from build123d import *

# Parameters (mm, degrees)
SKETCH_W        = 115
SKETCH_H        = 62
SKETCH_R        = 1.75
PAD_DEPTH       = 5
FILLET_R        = 1
FILLET001_R     = 1
FILLET002_R     = 3
PAD001_DEPTH    = 40
SKETCH002_W     = 95
SKETCH002_H     = 62
PAD002_DEPTH    = 3
FILLET003_R     = 3
FILLET004_R     = 1
SKETCH003_W     = 40
SKETCH003_H     = 15
POCKET_DEPTH    = 5
SKETCH004_R     = 1.75
POCKET001_DEPTH = 5
FILLET005_R     = 4
POCKET002_DEPTH = 5
SKETCH006_W     = 95
SKETCH006_H     = 43
POCKET003_DEPTH = 1
SKETCH007_W     = 95
SKETCH007_H     = 43
PAD003_DEPTH    = 1
PAD004_DEPTH    = 1
FILLET006_R     = 1


with BuildPart() as part:
    # Sketch → Pad (new body)
    with BuildSketch(Plane.XY):
        Rectangle(SKETCH_W, SKETCH_H)
        with Locations((-50, 22.5)):
            Circle(SKETCH_R, mode=Mode.SUBTRACT)
        with Locations((50, 22.5)):
            Circle(SKETCH_R, mode=Mode.SUBTRACT)
        with Locations((-50, -22.5)):
            Circle(SKETCH_R, mode=Mode.SUBTRACT)
        with Locations((50, -22.5)):
            Circle(SKETCH_R, mode=Mode.SUBTRACT)
        with BuildLine():
            ThreePointArc((-40.5, 15), (-42.62132, 14.12132), (-43.5, 12))
            Line((-43.5, -12), (-43.5, 12))
            ThreePointArc((-43.5, -12), (-42.62132, -14.12132), (-40.5, -15))
            Line((-40.5, -15), (-31.5, -15))
            ThreePointArc((-31.5, -15), (-29.37868, -14.12132), (-28.5, -12))
            Line((-28.5, 12), (-28.5, -12))
            ThreePointArc((-28.5, 12), (-29.37868, 14.12132), (-31.5, 15))
            Line((-40.5, 15), (-31.5, 15))
        make_face(mode=Mode.SUBTRACT)
    extrude(amount=PAD_DEPTH)

    # Fillet
    fillet_edges = [part.edges().sort_by_distance(p)[0] for p in [
        (-36, -15, 0),
        (-29.37868, -14.12132, 0),
        (-28.5, 0, 0),
        (-42.62132, -14.12132, 0),
        (-43.5, 0, 0),
        (-42.62132, 14.12132, 0),
        (-36, 15, 0),
        (-29.37868, 14.12132, 0),
    ]]
    fillet(fillet_edges, radius=FILLET_R)

    # Fillet001
    fillet001_edges = [part.edges().sort_by_distance(p)[0] for p in [
        (-43.5, 0, 5),
        (-42.62132, -14.12132, 5),
        (-36, -15, 5),
        (-29.37868, -14.12132, 5),
        (-28.5, 0, 5),
        (-29.37868, 14.12132, 5),
        (-36, 15, 5),
        (-42.62132, 14.12132, 5),
    ]]
    fillet(fillet001_edges, radius=FILLET001_R)

    # Fillet002
    fillet002_edges = [part.edges().sort_by_distance(p)[0] for p in [
        (-57.5, -31, 2.5),
        (-57.5, 31, 2.5),
        (57.5, -31, 2.5),
        (57.5, 31, 2.5),
    ]]
    fillet(fillet002_edges, radius=FILLET002_R)

    # Sketch001 (on Face1 of Fillet002) → Pad001 (join)
    with BuildSketch(Plane.XY.offset(5)):
        Polygon((-47.5, 31), (47.5, 31), (47.5, -31), (45.5, -31), (45.5, 29), (-45.5, 29), (-45.5, -31), (-47.5, -31), align=None)
    extrude(amount=PAD001_DEPTH)

    # Sketch002 (on Face15 of Pad001) → Pad002 (join)
    with BuildSketch(Plane.XY.offset(45)):
        Rectangle(SKETCH002_W, SKETCH002_H)
    extrude(amount=PAD002_DEPTH)

    # Fillet003
    fillet003_edges = [part.edges().sort_by_distance(p)[0] for p in [
        (-45.5, 29, 25),
        (45.5, 29, 25),
    ]]
    fillet(fillet003_edges, radius=FILLET003_R)

    # Fillet004
    fillet004_edges = [part.edges().sort_by_distance(p)[0] for p in [
        (-47.5, 31, 25),
        (-45.5, -2.5, 45),
        (-44.62132, 28.12132, 45),
        (0, 29, 45),
        (44.62132, 28.12132, 45),
        (45.5, -2.5, 45),
    ]]
    fillet(fillet004_edges, radius=FILLET004_R)

    # Sketch003 (on Face21 of Fillet004) → Pocket (cut)
    with BuildSketch(Plane(origin=(-47.5, 0, 0), x_dir=(0, -1, 0), z_dir=(-1, 0, 0))):
        with Locations((0, 15)):
            Rectangle(SKETCH003_W, SKETCH003_H)
    extrude(amount=-POCKET_DEPTH, mode=Mode.SUBTRACT)

    # Sketch004 → Pocket001 (cut)
    with BuildSketch(Plane.XY.offset(48)):
        with Locations((-40, -15)):
            Circle(SKETCH004_R)
        with Locations((-40, 15)):
            Circle(SKETCH004_R)
        with Locations((-10, 15)):
            Circle(SKETCH004_R)
        with Locations((10, 15)):
            Circle(SKETCH004_R)
        with Locations((40, 15)):
            Circle(SKETCH004_R)
        with Locations((40, -15)):
            Circle(SKETCH004_R)
        with Locations((10, -15)):
            Circle(SKETCH004_R)
        with Locations((-10, -15)):
            Circle(SKETCH004_R)
        with Locations((-42.5, -25)):
            Circle(SKETCH004_R)
        with Locations((-42.5, 25)):
            Circle(SKETCH004_R)
        with Locations((42.5, 25)):
            Circle(SKETCH004_R)
        with Locations((42.5, -25)):
            Circle(SKETCH004_R)
        with BuildLine():
            ThreePointArc((-17.5, 0), (-25, 7.5), (-32.5, 0))
            ThreePointArc((-32.5, 0), (-25, -7.5), (-17.5, 0))
        make_face()
        with BuildLine():
            ThreePointArc((32.5, 0), (25, 7.5), (17.5, 0))
            ThreePointArc((17.5, 0), (25, -7.5), (32.5, 0))
        make_face()
    extrude(amount=-POCKET001_DEPTH, mode=Mode.SUBTRACT)

    # Fillet005
    fillet005_edges = [part.edges().sort_by_distance(p)[0] for p in [
        (-46.5, 20, 22.5),
        (-46.5, 20, 7.5),
        (-46.5, -20, 22.5),
        (-46.5, -20, 7.5),
    ]]
    fillet(fillet005_edges, radius=FILLET005_R)

    # Sketch005 (on Face52 of Fillet005) → Pocket002 (cut)
    with BuildSketch(Plane(origin=(0, 0, 0), x_dir=(1, 0, 0), z_dir=(0, 0, -1))):
        with BuildLine():
            ThreePointArc((-40, 27), (-43.535534, 25.535534), (-45, 22))
            Line((-45, -22), (-45, 22))
            ThreePointArc((-45, -22), (-43.535534, -25.535534), (-40, -27))
            Line((40, -27), (-40, -27))
            ThreePointArc((40, -27), (43.535534, -25.535534), (45, -22))
            Line((45, 22), (45, -22))
            ThreePointArc((45, 22), (43.535534, 25.535534), (40, 27))
            Line((-40, 27), (40, 27))
        make_face()
    extrude(amount=-POCKET002_DEPTH, mode=Mode.SUBTRACT)

    # Sketch006 (on Face29 of Pocket002) → Pocket003 (cut)
    with BuildSketch(Plane.XZ.offset(31)):
        with Locations((0, 26.5)):
            Rectangle(SKETCH006_W, SKETCH006_H)
    extrude(amount=-POCKET003_DEPTH, mode=Mode.SUBTRACT)

    # Sketch007 (on Face4 of Pocket003) → Pad003 (join)
    with BuildSketch(Plane.XZ.offset(30)):
        with Locations((0, 26.5)):
            Rectangle(SKETCH007_W, SKETCH007_H)
    extrude(amount=PAD003_DEPTH)

    # Pad003 Face4 → Pad004 (add)
    with BuildSketch(Plane(origin=(0, -30, 24.997668), x_dir=(1, 0, 0), z_dir=(0, 1, 0))):
        with BuildLine():
            Line((45.5, -19.002332), (45.5, 19.997668))
            Line((45.5, 19.997668), (-45.5, 19.997668))
            Line((-45.5, 19.997668), (-45.5, -19.002332))
            ThreePointArc((-45.5, -19.002332), (-45.207107, -19.709439), (-44.5, -20.002332))
            Line((-44.5, -20.002332), (44.5, -20.002332))
            ThreePointArc((44.5, -20.002332), (45.207107, -19.709439), (45.5, -19.002332))
        make_face()
    extrude(amount=PAD004_DEPTH)

    # Fillet006
    fillet006_edges = [part.edges().sort_by_distance(p)[0] for p in [
        (0, -29, 45),
    ]]
    fillet(fillet006_edges, radius=FILLET006_R)


solid = part.part
Check sheet for the modelled part. Datum: model origin and axes. Units: mm. A direction names the side the tool comes from. Round coordinates to 2 decimals unless told otherwise and drop trailing zeros. Write each loop counter-clockwise with the first axis right and the second up, starting at its lowest first coordinate (ties: lowest second). Pieces come first, ordered by that corner, then holes. Notation, with made-up numbers: (3, -24.5) - (32, -24.5) arc R10 cw to (32, -12.5) - close; hole circle Ø1 at (41.5, 30.5). An arc over 180 degrees is marked (long way). Return JSON: item names as keys, results as strings.
Q1. Draft check along Y on faces 1 (the flat face through (47.5, 0, 26)), 2 (the flat face through (-1, 31, 24)), 3 (the cylindrical face through (-41.6, -23.5, 46.5)). Enter one of: released by +Y, released by -Y, zero draft, split by the parting line, or undercut.
Returned:
{"face 1": "zero draft", "face 2": "released by +Y", "face 3": "undercut"}
Q2. Depth check by flat-ended pin: P1, Ø12, axis at x = -53, y = 6, coming from the +Z side; P2, Ø5.5, axis at x = -10, y = 15, coming from the -Z side; P3, Ø3, axis at x = 54.5, y = 11.5, coming from the +Z side; P4, Ø8, axis at y = 9.5, z = 16, coming from the -X side. Enter the tip coordinate at first touch or a pass-through.
Returned:
{"P1": "stops at z = 48", "P2": "stops at z = 45", "P3": "stops at z = 5", "P4": "stops at x = 45.5"}
Q3. Access from +Z, -Z, +X, -X, +Y, -Y to the whole of each face (thin tool, end or side, straight path). Record for faces 4 (the cylindrical face through (-44, 25, 2)), 5 (the cylindrical face through (-41.6, 26.5, 46.5)), 6 (the flat face through (-45.5, -1, 29)).
Returned:
{"face 4": "-Z", "face 5": "+Z", "face 6": "none"}
Q4. Scan lines: L1, parallel to Y at x = -50, z = 1; L2, parallel to Y at x = -42.5, z = 46.55; L3, parallel to X at y = -16, z = 32. Record each from-to range of solid material in increasing order. Write a range as from..to.
Returned:
{"L1": "y = -31..-24.25, -20.75..20.75, 24.25..31", "L2": "y = -31..-26.75, -23.25..23.25, 26.75..31", "L3": "x = -47.5..-45.5, 45.5..47.5"}
Q5. Cross-section at B-B (y = -9). Record the boundary of the cut face in (x, z).
Returned:
{"outline": "(-57.5, 0) - (-45, 0) - (-45, 5) - (-45.5, 5) - (-45.5, 7.5) - (-47.5, 7.5) - (-47.5, 5) - (-57.5, 5) - close; (-47.5, 22.5) - (-45.5, 22.5) - (-45.5, 44) arc R1 cw to (-44.5, 45) - (44.5, 45) arc R1 cw to (45.5, 44) - (45.5, 5) - (45, 5) - (45, 0) - (57.5, 0) - (57.5, 5) - (47.5, 5) - (47.5, 48) - (-47.5, 48) - close"}
Q6. Cross-section at C-C (z = 37.5). Record the boundary of the cut face in (x, y).
Returned:
{"outline": "(-47.5, -31) - (47.5, -31) - (47.5, 31) - (-46.5, 31) arc R1 ccw to (-47.5, 30) - close; hole (-45.5, -28) arc R1 ccw to (-44.5, -29) - (44.5, -29) arc R1 ccw to (45.5, -28) - (45.5, 26) arc R3 ccw to (42.5, 29) - (-42.5, 29) arc R3 ccw to (-45.5, 26) - close"}
Q7. Cross-section at A-A (x = -50). Record the boundary of the cut face in (y, z), then the cut area to 3 significant figures.
Returned:
{"outline": "(-31, 0) - (-24.25, 0) - (-24.25, 5) - (-31, 5) - close; (-20.75, 0) - (20.75, 0) - (20.75, 5) - (-20.75, 5) - close; (24.25, 0) - (31, 0) - (31, 5) - (24.25, 5) - close", "area": "275 mm²"}
Q8. Cross-section at D-D (x = 25). Record the boundary of the cut face in (y, z).
Returned:
{"outline": "(-31, 0) - (-27, 0) - (-27, 5) - (-29, 5) - (-29, 44) arc R1 cw to (-28, 45) - (-7.5, 45) - (-7.5, 48) - (-31, 48) - close; (7.5, 45) - (28, 45) arc R1 cw to (29, 44) - (29, 5) - (27, 5) - (27, 0) - (31, 0) - (31, 48) - (7.5, 48) - close"}
